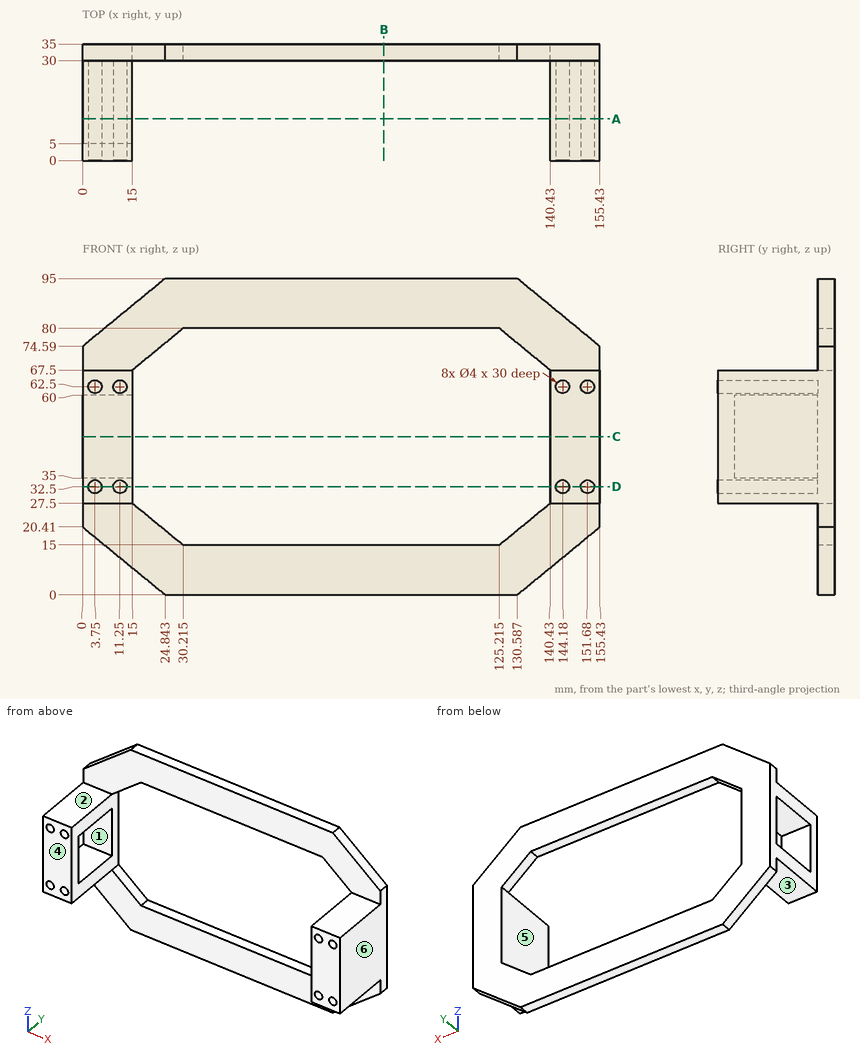
The drawing under review shows one solid part. Ordinate dimensions are in mm from its lowest x, y, z. A direction names the side the tool comes from. Round coordinates to 2 decimals unless told otherwise and drop trailing zeros. Write each loop counter-clockwise with the first axis right and the second up, starting at its lowest first coordinate (ties: lowest second). Pieces come first, ordered by that corner, then holes. Notation, with made-up numbers: (47, 32.25) - (73, 32.25) arc R8 ccw to (73, 41.25) - close; hole circle Ø1 at (69.5, 0.5). An arc over 180 degrees is marked (long way). One line per question, with ' | ' between items.
Item 1: To check wall thickness, follow probe 1 along X at (y, z) = (9.25, 32.5); probe 2 along Z at (x, y) = (11, 18) (1 decimal); probe 3 along Z at (x, y) = (144, 8). State the ranges of each line that lie inside material, in increasing order.
Resolved:
probe 1: x = 0 to 1.75, 5.75 to 9.25, 13.25 to 15, 140.43 to 142.18, 146.18 to 149.68, 153.68 to 155.43 | probe 2: z = 27.5 to 30.5, 34.5 to 35, 60 to 60.5, 64.5 to 67.5 | probe 3: z = 27.5 to 30.51, 34.49 to 60.51, 64.49 to 67.5
Item 2: Add section A-A, the plane y = 12.5. State how many separate pieces and enclosed holes the cut face has.
Resolved:
separate pieces: 3 | enclosed holes: 8
Item 3: The part is to be moulded in two halves that separate along X. For the marked faces 4, 5 and 6, say which applies: pulls with the +X half, pulls with the -X half, needs draft (parallel to the pull), parting line crosses it, or undercut.
Resolved:
face 4: needs draft | face 5: undercut | face 6: pulls with the +X half
Item 4: Add section B-B, the plane x = 90.5. Give the boundary of the cut face in (y, z).
Resolved:
outline: (30, 0) - (35, 0) - (35, 15) - (30, 15) - close; (30, 80) - (35, 80) - (35, 95) - (30, 95) - close
Item 5: For the marked faces 1, 2 and 3, list the 3-axis set-ups (+Z, -Z, +X, -X, +Y, -Y) from which the entire face can be reached by the end or side of a thin tool; tool diameter is ignored.
Resolved:
face 1: -X | face 2: +Z, +X, -X, -Y | face 3: -Z, +X, -X, -Y
Item 6: For P1, Ø12, axis at x = 150, y = 16, coming from the -Z side; P2, Ø2, axis at x = 11, z = 33.5, coming from the -Y side; P3, Ø16.5, axis at x = 147, y = 9.5, coming from the +Z side; P4, Ø22, axis at x = 112, z = 79, coming from the -Y side, all flat-tipped, find the tip position at first contact; note any pin that passes through.
Resolved:
P1: stops at z = 27.5 | P2: stops at y = 0 | P3: stops at z = 67.5 | P4: stops at y = 30
Item 7: Add section D-D, the plane z = 32.5. Give the boundary of the cut face in (x, y), then the cut area to 3 significant figures.
Resolved:
outline: (0, 0) - (1.75, 0) - (1.75, 30) - (5.75, 30) - (5.75, 0) - (9.25, 0) - (9.25, 30) - (13.25, 30) - (13.25, 0) - (15, 0) - (15, 35) - (0, 35) - close; (140.43, 0) - (142.18, 0) - (142.18, 30) - (146.18, 30) - (146.18, 0) - (149.68, 0) - (149.68, 30) - (153.68, 30) - (153.68, 0) - (155.43, 0) - (155.43, 35) - (140.43, 35) - close | area: 570 mm2
Item 8: Add section C-C, the plane z = 47.5. Give the boundary of the cut face in (x, y), then the cut area to 3 significant figures.
Resolved:
outline: (0, 0) - (15, 0) - (15, 5) - (0, 5) - close; (0, 30) - (15, 30) - (15, 35) - (0, 35) - close; (140.43, 0) - (155.43, 0) - (155.43, 35) - (140.43, 35) - close | area: 675 mm2
